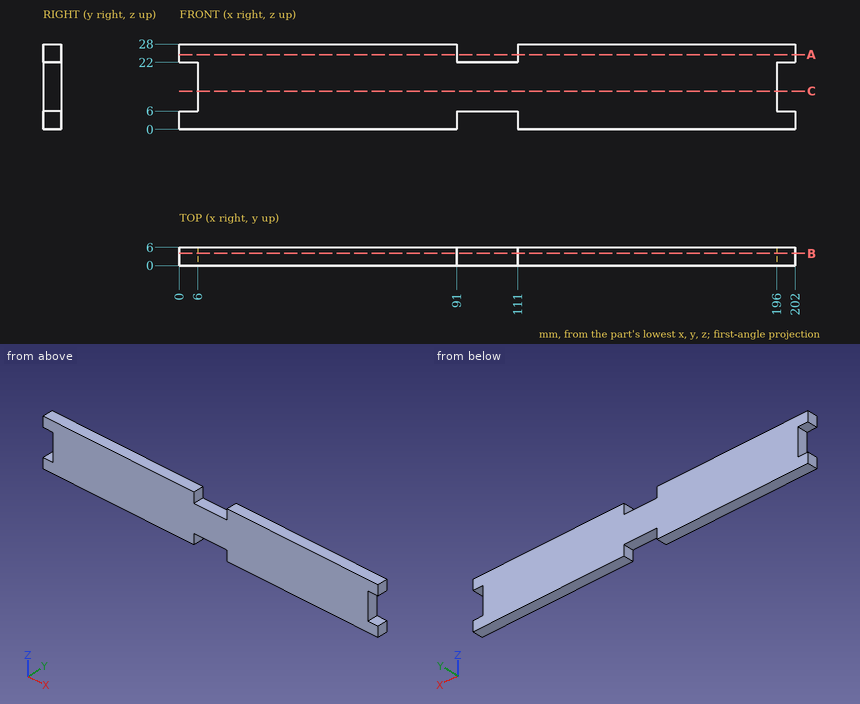
The drawing under review shows one solid part. Ordinate dimensions are in mm from its lowest x, y, z. Round coordinates to 2 decimals unless told otherwise and drop trailing zeros. Order: outer loops, then holes, each group sorted by start corner. A loop starts at its lowest first (then second) coordinate and runs counter-clockwise, first axis right, second up. Notation, with made-up numbers: (67.5, -0.5) -> (117.5, -0.5) arc R19 cw to (117.5, 31.5) -> close; hole circle Ø1 at (46, 17.5). An arc over 180 degrees is marked (long way). Return JSON: item names as keys, results as strings.
1. Take a section at B-B (y = 4.05). Write out the cut boundary in (x, z), then the cut area to 3 significant figures.
Answer block:
{"outline": "(0, 0) -> (91, 0) -> (91, 6) -> (111, 6) -> (111, 0) -> (202, 0) -> (202, 6) -> (196, 6) -> (196, 22) -> (202, 22) -> (202, 28) -> (111, 28) -> (111, 22) -> (91, 22) -> (91, 28) -> (0, 28) -> (0, 22) -> (6, 22) -> (6, 6) -> (0, 6) -> close", "area": "5,220 mm²"}
2. Insertion check: P1, Ø1.8, axis at y = 4, z = 10.5, coming from the +X side; P2, Ø1.8, axis at x = 101, y = 2, coming from the +Z side; P3, Ø3, axis at y = 4, z = 11, coming from the -X side. Each pin has a flat end and moves straight along its axis. Give the tip position at first contact, or say it passes through.
Answer block:
{"P1": "stops at x = 196", "P2": "stops at z = 22", "P3": "stops at x = 6"}
3. Take a section at A-A (z = 24.5). Write out the cut boundary in (x, y).
Answer block:
{"outline": "(0, 0) -> (91, 0) -> (91, 6) -> (0, 6) -> close; (111, 0) -> (202, 0) -> (202, 6) -> (111, 6) -> close"}
4. For L1, parallel to X at y = 3.55, z = 3.75; L2, parallel to X at y = 3.35, z = 17.25; L3, parallel to Z at x = 99, y = 3.25, list the stretches that pass through material, from the lowest coordinate up. Write a range as [from, to].
Answer block:
{"L1": "x = [0, 91], [111, 202]", "L2": "x = [6, 196]", "L3": "z = [6, 22]"}
5. Take a section at C-C (z = 12.5). Write out the cut boundary in (x, y), then the cut area to 3 significant figures.
Answer block:
{"outline": "(6, 0) -> (196, 0) -> (196, 6) -> (6, 6) -> close", "area": "1,140 mm²"}
